```python
from build123d import *

# Parameters (mm, degrees)
BOSS_EXTRUDE1_DEPTH = 5
BOSS_EXTRUDE2_DEPTH = 2
SKETCH4_W           = 24
SKETCH4_H           = 3
BOSS_EXTRUDE3_DEPTH = 49
CUT_EXTRUDE1_REACH  = 10.25
SKETCH5_R           = 1.75
SKETCH5_W           = 14
SKETCH5_H           = 24
SKETCH6_R           = 3.25
SKETCH6_R_2         = 1.75
BOSS_EXTRUDE4_DEPTH = 3
FILLET1_R           = 2


with BuildPart() as part:
    # Sketch1 → Boss-Extrude1 (new body)
    with BuildSketch(Plane(origin=(0, 0, 0), x_dir=(1, 0, 0), z_dir=(0, 1, 0))):
        with BuildLine():
            Line((-18.25, 6.75), (18.25, 6.75))
            ThreePointArc((18.25, 6.75), (20.371320344, 5.871320344), (21.25, 3.75))
            Line((21.25, 3.75), (21.25, -3.75))
            ThreePointArc((21.25, -3.75), (20.371320344, -5.871320344), (18.25, -6.75))
            Line((18.25, -6.75), (-18.25, -6.75))
            ThreePointArc((-18.25, -6.75), (-20.371320344, -5.871320344), (-21.25, -3.75))
            Line((-21.25, -3.75), (-21.25, 3.75))
            ThreePointArc((-21.25, 3.75), (-20.371320344, 5.871320344), (-18.25, 6.75))
        make_face()
        with BuildLine():
            Line((16.260111444, 2.189943648), (0.716289014, 3.681276533))
            ThreePointArc((0.716289014, 3.681276533), (0, 3.715559552), (-0.716289014, 3.681276533))
            Line((-0.716289014, 3.681276533), (-16.260111444, 2.189943648))
            ThreePointArc((-16.260111444, 2.189943648), (-18.25, 0), (-16.260111444, -2.189943648))
            Line((-16.260111444, -2.189943648), (-0.716289014, -3.681276533))
            ThreePointArc((-0.716289014, -3.681276533), (0, -3.715559552), (0.716289014, -3.681276533))
            Line((0.716289014, -3.681276533), (16.260111444, -2.189943648))
            ThreePointArc((16.260111444, -2.189943648), (18.25, 0), (16.260111444, 2.189943648))
        make_face(mode=Mode.SUBTRACT)
    extrude(amount=BOSS_EXTRUDE1_DEPTH)

    # Sketch2 → Boss-Extrude2 (add)
    with BuildSketch(Plane.XZ):
        with BuildLine():
            Line((-16.260111444, 2.189943648), (-6, 3.174337395))
            Line((-6, 3.174337395), (-6, -3.174337395))
            Line((-6, -3.174337395), (-16.260111444, -2.189943648))
            ThreePointArc((-16.260111444, -2.189943648), (-18.25, 0), (-16.260111444, 2.189943648))
        make_face()
        with BuildLine():
            Line((6, -3.174337395), (16.260111444, -2.189943648))
            ThreePointArc((16.260111444, -2.189943648), (18.25, 0), (16.260111444, 2.189943648))
            Line((16.260111444, 2.189943648), (6, 3.174337395))
            Line((6, 3.174337395), (6, -3.174337395))
        make_face()
    extrude(amount=-BOSS_EXTRUDE2_DEPTH)

    # Sketch4 → Boss-Extrude3 (add)
    with BuildSketch(Plane(origin=(24.5, 24.5, 0), x_dir=(0, -1, 0), z_dir=(-1, 0, 0))):
        with Locations((36.5, 0)):
            Rectangle(SKETCH4_W, SKETCH4_H)
    extrude(amount=BOSS_EXTRUDE3_DEPTH)

    # Sketch5 → Cut-Extrude1 (cut, up to next)
    with BuildSketch(Plane(origin=(0, 0, -1.5), x_dir=(-1, 0, 0), z_dir=(0, 0, -1)), mode=Mode.PRIVATE) as cut_extrude1_sk1:
        with Locations((20.35, -19.85)):
            Circle(SKETCH5_R)
    cut_extrude1_tool1 = extrude(cut_extrude1_sk1.sketch, amount=-CUT_EXTRUDE1_REACH, mode=Mode.PRIVATE) & part.part
    add(cut_extrude1_tool1.solids().sort_by_distance((-20.35, -19.85, -1.5))[0], mode=Mode.SUBTRACT)
    # Sketch5 → Cut-Extrude1 (cut, up to next)
    with BuildSketch(Plane(origin=(0, 0, -1.5), x_dir=(-1, 0, 0), z_dir=(0, 0, -1)), mode=Mode.PRIVATE) as cut_extrude1_sk2:
        with Locations((-20.35, -19.85)):
            Circle(SKETCH5_R)
    cut_extrude1_tool2 = extrude(cut_extrude1_sk2.sketch, amount=-CUT_EXTRUDE1_REACH, mode=Mode.PRIVATE) & part.part
    add(cut_extrude1_tool2.solids().sort_by_distance((20.35, -19.85, -1.5))[0], mode=Mode.SUBTRACT)
    # Sketch5 → Cut-Extrude1 (cut, up to next)
    with BuildSketch(Plane(origin=(0, 0, -1.5), x_dir=(-1, 0, 0), z_dir=(0, 0, -1)), mode=Mode.PRIVATE) as cut_extrude1_sk3:
        with Locations((-20.35, -4.15)):
            Circle(SKETCH5_R)
    cut_extrude1_tool3 = extrude(cut_extrude1_sk3.sketch, amount=-CUT_EXTRUDE1_REACH, mode=Mode.PRIVATE) & part.part
    add(cut_extrude1_tool3.solids().sort_by_distance((20.35, -4.15, -1.5))[0], mode=Mode.SUBTRACT)
    # Sketch5 → Cut-Extrude1 (cut, up to next)
    with BuildSketch(Plane(origin=(0, 0, -1.5), x_dir=(-1, 0, 0), z_dir=(0, 0, -1)), mode=Mode.PRIVATE) as cut_extrude1_sk4:
        with Locations((20.35, -4.15)):
            Circle(SKETCH5_R)
    cut_extrude1_tool4 = extrude(cut_extrude1_sk4.sketch, amount=-CUT_EXTRUDE1_REACH, mode=Mode.PRIVATE) & part.part
    add(cut_extrude1_tool4.solids().sort_by_distance((-20.35, -4.15, -1.5))[0], mode=Mode.SUBTRACT)
    # Sketch5 → Cut-Extrude1 (cut, up to next)
    with BuildSketch(Plane(origin=(0, 0, -1.5), x_dir=(-1, 0, 0), z_dir=(0, 0, -1)), mode=Mode.PRIVATE) as cut_extrude1_sk5:
        with Locations((0, -12)):
            Rectangle(SKETCH5_W, SKETCH5_H)
    cut_extrude1_tool5 = extrude(cut_extrude1_sk5.sketch, amount=-CUT_EXTRUDE1_REACH, mode=Mode.PRIVATE) & part.part
    add(cut_extrude1_tool5.solids().sort_by_distance((0, -12, -1.5))[0], mode=Mode.SUBTRACT)

    # Sketch6 → Boss-Extrude4 (add)
    with BuildSketch(Plane(origin=(0, 0, -1.5), x_dir=(-1, 0, 0), z_dir=(0, 0, -1))):
        with Locations((-20.35, -4.15)):
            Circle(SKETCH6_R)
        with Locations((-20.35, -4.15)):
            Circle(SKETCH6_R_2, mode=Mode.SUBTRACT)
        with Locations((20.35, -4.15)):
            Circle(SKETCH6_R)
        with Locations((20.35, -4.15)):
            Circle(SKETCH6_R_2, mode=Mode.SUBTRACT)
        with Locations((20.35, -19.85)):
            Circle(SKETCH6_R)
        with Locations((20.35, -19.85)):
            Circle(SKETCH6_R_2, mode=Mode.SUBTRACT)
        with Locations((-20.35, -19.85)):
            Circle(SKETCH6_R)
        with Locations((-20.35, -19.85)):
            Circle(SKETCH6_R_2, mode=Mode.SUBTRACT)
    extrude(amount=BOSS_EXTRUDE4_DEPTH)

    # Fillet1
    fillet1_edges = [part.edges().sort_by_distance(p)[0] for p in [
        (24.5, 0, 0),
        (24.5, -24, 0),
        (-24.5, 0, 0),
        (-24.5, -24, 0),
    ]]
    fillet(fillet1_edges, radius=FILLET1_R)


solid = part.part
```
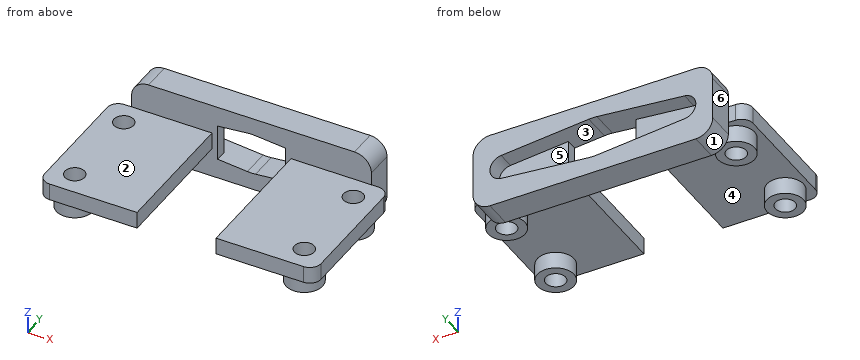
Check sheet for the modelled part. Datum: model origin and axes. Units: mm. Face numbers are marked on the shaded views. A direction names the side the tool comes from. Coordinates: 2 decimals unless noted, no trailing zeros. Write each loop counter-clockwise with the first axis right and the second up, starting at its lowest first coordinate (ties: lowest second). Pieces come first, ordered by that corner, then holes. Notation, with made-up numbers: (53.5, 34.5) - (79.5, 34.5) arc R30 cw to (79.5, 60.5) - close; hole circle Ø7 at (57, 82). An arc over 180 degrees is marked (long way). One line per question, with ' | ' between items.
Item 1: Thickness scan on line 1 (Y direction, x = -20.35, z = -3.6); line 2 (Y direction, x = -20.35, z = -0.6); line 3 (Z direction, x = 13.5, y = -2). Record the ranges inside material, lowest first. Write a range as [from, to].
Determined:
line 1: y = [-23.1, -21.6], [-18.1, -16.6], [-7.4, -5.9], [-2.4, -0.9], [0, 5] | line 2: y = [-24, -21.6], [-18.1, -5.9], [-2.4, 5] | line 3: z = [-1.5, 1.5]
Item 2: Sectioned sample at A-A on y = -4.15. Record the boundary of the cut face in (x, z).
Determined:
outline: (-24.5, -1.5) - (-23.6, -1.5) - (-23.6, -4.5) - (-22.1, -4.5) - (-22.1, 1.5) - (-24.5, 1.5) - close; (-18.6, -4.5) - (-17.1, -4.5) - (-17.1, -1.5) - (-7, -1.5) - (-7, 1.5) - (-18.6, 1.5) - close; (7, -1.5) - (17.1, -1.5) - (17.1, -4.5) - (18.6, -4.5) - (18.6, 1.5) - (7, 1.5) - close; (22.1, -4.5) - (23.6, -4.5) - (23.6, -1.5) - (24.5, -1.5) - (24.5, 1.5) - (22.1, 1.5) - close
Item 3: Sectioned sample at B-B on z = -0.25. Record the boundary of the cut face in (x, y), plus the area to 3 significant figures.
Determined:
outline: (-24.5, -22) arc R2 ccw to (-22.5, -24) - (-7, -24) - (-7, 0) - (-6, 0) - (-6, 2) - (-18.24, 2) - (-18.24, 5) - (-21.25, 5) - (-21.25, 0) - (-22.5, 0) arc R2 ccw to (-24.5, -2) - close; (6, 0) - (7, 0) - (7, -24) - (22.5, -24) arc R2 ccw to (24.5, -22) - (24.5, -2) arc R2 ccw to (22.5, 0) - (21.25, 0) - (21.25, 5) - (18.24, 5) - (18.24, 2) - (6, 2) - close; hole circle Ø3.5 at (-20.35, -19.85); hole circle Ø3.5 at (-20.35, -4.15); hole circle Ø3.5 at (20.35, -19.85); hole circle Ø3.5 at (20.35, -4.15) | area: 877 mm2
Item 4: Gauge pin test, flat ends, axial feed: P1, Ø0.6, axis at y = 0.5, z = -0.5, coming from the +X side; P2, Ø5, axis at x = 13, y = -8.5, coming from the -Z side; P3, Ø5.5, axis at x = 20.35, y = -4.15, coming from the +Z side; P4, Ø3, axis at x = -20.35, y = -4.15, coming from the +Z side. Record the tip position at first contact, or that the pin passes through.
Determined:
P1: stops at x = 21.25 | P2: stops at z = -1.5 | P3: stops at z = 1.5 | P4: passes through
Item 5: Sectioned sample at D-D on x = -10. Record the boundary of the cut face in (y, z), plus the area to 3 significant figures.
Determined:
outline: (-24, -1.5) - (0, -1.5) - (0, -6.75) - (5, -6.75) - (5, -2.79) - (2, -2.79) - (2, 2.79) - (5, 2.79) - (5, 6.75) - (0, 6.75) - (0, 1.5) - (-24, 1.5) - close | area: 123 mm2
Item 6: Sectioned sample at C-C on x = 20.35. Record the boundary of the cut face in (y, z), plus the area to 3 significant figures.
Determined:
outline: (-24, -1.5) - (-23.1, -1.5) - (-23.1, -4.5) - (-21.6, -4.5) - (-21.6, 1.5) - (-24, 1.5) - close; (-18.1, -4.5) - (-16.6, -4.5) - (-16.6, -1.5) - (-7.4, -1.5) - (-7.4, -4.5) - (-5.9, -4.5) - (-5.9, 1.5) - (-18.1, 1.5) - close; (-2.4, -4.5) - (-0.9, -4.5) - (-0.9, -1.5) - (0, -1.5) - (0, -5.89) - (5, -5.89) - (5, 5.89) - (0, 5.89) - (0, 1.5) - (-2.4, 1.5) - close | area: 128 mm2
Item 7: Mould release check, pull along X, two halves, no side actions. Record for the marked faces 1, 2 and 3: pulls with the +X half, pulls with the -X half, needs draft (parallel to the pull), parting line crosses it, or undercut.
Determined:
face 1: pulls with the -X half | face 2: needs draft | face 3: undercut
Item 8: Access from +Z, -Z, +X, -X, +Y, -Y to the whole of each face (thin tool, end or side, straight path). Record for the marked faces 4, 5 and 6.
Determined:
face 4: -Z | face 5: +Y | face 6: +Z, -Z, -X, +Y
